from build123d import *

# Parameters (mm, degrees)
BOSS_EXTRUDE1_DEPTH = 19.05
SKETCH2_R           = 3.175
CUT_EXTRUDE1_DEPTH  = 169.2497345
SKETCH4_W           = 25.654
SKETCH4_H           = 25.654
CUT_EXTRUDE2_DEPTH  = 169.2497345


with BuildPart() as part:
    # Sketch1 → Boss-Extrude1 (new body)
    with BuildSketch(Plane(origin=(0, 0, 0), x_dir=(1, 0, 0), z_dir=(0, 1, 0))):
        with BuildLine():
            Line((41.324442937, 92.816218496), (0, 0))
            Line((0, 0), (0, 101.6))
            Line((0, 101.6), (-21.123827787, 99.379796235))
            Line((-21.123827787, 99.379796235), (-26.134113546, 108.80277326))
            ThreePointArc((-26.134113546, 108.80277326), (-30.395027803, 112.639317689), (-36.125160716, 112.83941834))
            Line((-36.125160716, 112.83941834), (-37.099477034, 112.522843778))
            ThreePointArc((-37.099477034, 112.522843778), (-41.617635729, 108.992871331), (-42.809723539, 103.384539126))
            Line((-42.809723539, 103.384539126), (-41.324442937, 92.816218496))
            Line((-41.324442937, 92.816218496), (-59.718981633, 82.196126628))
            Line((-59.718981633, 82.196126628), (-68.128775472, 88.766577677))
            ThreePointArc((-68.128775472, 88.766577677), (-73.58177754, 90.538365452), (-78.897902701, 88.390511467))
            Line((-78.897902701, 88.390511467), (-79.659222473, 87.705016066))
            ThreePointArc((-79.659222473, 87.705016066), (-82.350996682, 82.642525071), (-81.158908872, 77.034192866))
            Line((-81.158908872, 77.034192866), (-75.503514269, 67.983669606))
            Line((-75.503514269, 67.983669606), (-87.988181024, 50.8))
            Line((-87.988181024, 50.8), (-98.343353189, 53.381834395))
            ThreePointArc((-98.343353189, 53.381834395), (-104.04556947, 52.782507313), (-108.028480544, 48.658082159))
            Line((-108.028480544, 48.658082159), (-108.445164665, 47.722194301))
            ThreePointArc((-108.445164665, 47.722194301), (-108.845122174, 42.002535442), (-105.474981556, 37.363934825))
            Line((-105.474981556, 37.363934825), (-96.627342056, 31.396126628))
            Line((-96.627342056, 31.396126628), (-101.043424569, 10.620091868))
            Line((-101.043424569, 10.620091868), (-111.553471718, 8.766886987))
            ThreePointArc((-111.553471718, 8.766886987), (-116.518937215, 5.900074146), (-118.479952693, 0.512228401))
            Line((-118.479952693, 0.512228401), (-118.479952693, -0.512228401))
            ThreePointArc((-118.479952693, -0.512228401), (-116.518937215, -5.900074146), (-111.553471718, -8.766886987))
            Line((-111.553471718, -8.766886987), (-101.043424569, -10.620091868))
            Line((-101.043424569, -10.620091868), (-96.627342056, -31.396126628))
            Line((-96.627342056, -31.396126628), (-105.474981556, -37.363934825))
            ThreePointArc((-105.474981556, -37.363934825), (-108.845122174, -42.002535442), (-108.445164665, -47.722194301))
            Line((-108.445164665, -47.722194301), (-108.028480544, -48.658082159))
            ThreePointArc((-108.028480544, -48.658082159), (-104.04556947, -52.782507313), (-98.343353189, -53.381834395))
            Line((-98.343353189, -53.381834395), (-87.988181024, -50.8))
            Line((-87.988181024, -50.8), (-75.503514269, -67.983669606))
            Line((-75.503514269, -67.983669606), (-81.158908872, -77.034192866))
            ThreePointArc((-81.158908872, -77.034192866), (-82.350996682, -82.642525071), (-79.659222473, -87.705016066))
            Line((-79.659222473, -87.705016066), (-78.897902701, -88.390511467))
            ThreePointArc((-78.897902701, -88.390511467), (-73.58177754, -90.538365452), (-68.128775472, -88.766577677))
            Line((-68.128775472, -88.766577677), (-59.718981633, -82.196126628))
            Line((-59.718981633, -82.196126628), (-41.324442937, -92.816218496))
            Line((-41.324442937, -92.816218496), (-42.809723539, -103.384539126))
            ThreePointArc((-42.809723539, -103.384539126), (-41.617635729, -108.992871331), (-37.099477034, -112.522843778))
            Line((-37.099477034, -112.522843778), (-36.125160716, -112.83941834))
            ThreePointArc((-36.125160716, -112.83941834), (-30.395027803, -112.639317689), (-26.134113546, -108.80277326))
            Line((-26.134113546, -108.80277326), (-21.123827787, -99.379796235))
            Line((-21.123827787, -99.379796235), (0, -101.6))
            Line((0, -101.6), (2.941651908, -111.858759352))
            ThreePointArc((2.941651908, -111.858759352), (6.311792526, -116.497359969), (11.875105022, -117.884449563))
            Line((11.875105022, -117.884449563), (12.893949744, -117.777364667))
            ThreePointArc((12.893949744, -117.777364667), (18.047298371, -115.263908602), (20.379374034, -110.025980903))
            Line((20.379374034, -110.025980903), (21.123827787, -99.379796235))
            Line((21.123827787, -99.379796235), (41.324442937, -92.816218496))
            Line((41.324442937, -92.816218496), (48.184389016, -100.991583882))
            ThreePointArc((48.184389016, -100.991583882), (53.149854513, -103.858396723), (58.796373538, -102.862763072))
            Line((58.796373538, -102.862763072), (59.683579155, -102.35053467))
            ThreePointArc((59.683579155, -102.35053467), (63.369082702, -97.958322577), (63.369082702, -92.224696894))
            Line((63.369082702, -92.224696894), (59.718981633, -82.196126628))
            Line((59.718981633, -82.196126628), (75.503514269, -67.983669606))
            Line((75.503514269, -67.983669606), (85.095607522, -72.662046078))
            ThreePointArc((85.095607522, -72.662046078), (90.797823803, -73.26137316), (95.551214921, -70.055170367))
            Line((95.551214921, -70.055170367), (96.153375521, -69.226367403))
            ThreePointArc((96.153375521, -69.226367403), (97.733776944, -63.714852656), (95.401701281, -58.476924957))
            Line((95.401701281, -58.476924957), (87.988181024, -50.8))
            Line((87.988181024, -50.8), (96.627342056, -31.396126628))
            Line((96.627342056, -31.396126628), (107.293022418, -31.768580394))
            ThreePointArc((107.293022418, -31.768580394), (112.746024485, -29.996792619), (115.784383188, -25.134402274))
            Line((115.784383188, -25.134402274), (115.997379734, -24.13233231))
            ThreePointArc((115.997379734, -24.13233231), (115.199413268, -18.454505879), (110.938499011, -14.617961449))
            Line((110.938499011, -14.617961449), (101.043424569, -10.620091868))
            Line((101.043424569, -10.620091868), (101.043424569, 10.620091868))
            Line((101.043424569, 10.620091868), (110.938499011, 14.617961449))
            ThreePointArc((110.938499011, 14.617961449), (115.199413268, 18.454505879), (115.997379734, 24.13233231))
            Line((115.997379734, 24.13233231), (115.784383188, 25.134402274))
            ThreePointArc((115.784383188, 25.134402274), (112.746024485, 29.996792619), (107.293022418, 31.768580394))
            Line((107.293022418, 31.768580394), (96.627342056, 31.396126628))
            Line((96.627342056, 31.396126628), (87.988181024, 50.8))
            Line((87.988181024, 50.8), (95.401701281, 58.476924957))
            ThreePointArc((95.401701281, 58.476924957), (97.733776944, 63.714852656), (96.153375521, 69.226367403))
            Line((96.153375521, 69.226367403), (95.551214921, 70.055170367))
            ThreePointArc((95.551214921, 70.055170367), (90.797823803, 73.26137316), (85.095607522, 72.662046078))
            Line((85.095607522, 72.662046078), (75.503514269, 67.983669606))
            Line((75.503514269, 67.983669606), (59.718981633, 82.196126628))
            Line((59.718981633, 82.196126628), (63.369082702, 92.224696894))
            ThreePointArc((63.369082702, 92.224696894), (63.369082702, 97.958322577), (59.683579155, 102.35053467))
            Line((59.683579155, 102.35053467), (58.796373538, 102.862763072))
            ThreePointArc((58.796373538, 102.862763072), (53.149854513, 103.858396723), (48.184389016, 100.991583882))
            Line((48.184389016, 100.991583882), (41.324442937, 92.816218496))
        make_face()
        with BuildLine():
            Line((0, 101.6), (0, 0))
            Line((0, 0), (21.123827787, 99.379796235))
            Line((21.123827787, 99.379796235), (20.379374034, 110.025980903))
            ThreePointArc((20.379374034, 110.025980903), (18.047298371, 115.263908602), (12.893949744, 117.777364667))
            Line((12.893949744, 117.777364667), (11.875105022, 117.884449563))
            ThreePointArc((11.875105022, 117.884449563), (6.311792526, 116.497359969), (2.941651908, 111.858759352))
            Line((2.941651908, 111.858759352), (0, 101.6))
        make_face()
        Polygon((21.123827787, 99.379796235), (0, 0), (41.324442937, 92.816218496), align=None)
    extrude(amount=BOSS_EXTRUDE1_DEPTH)

    # Sketch2 → Cut-Extrude1 (cut, through all)
    with BuildSketch(Plane(origin=(0, 19.05, 0), x_dir=(1, 0, 0), z_dir=(0, 1, 0))):
        with Locations(Location((0, 0, 0), (0, 0, 270))):
            Circle(SKETCH2_R)
    extrude(amount=-CUT_EXTRUDE1_DEPTH, mode=Mode.SUBTRACT)

    # Sketch4 → Cut-Extrude2 (cut, through all)
    with BuildSketch(Plane(origin=(0, 19.05, 0), x_dir=(1, 0, 0), z_dir=(0, 1, 0))):
        Rectangle(SKETCH4_W, SKETCH4_H)
    extrude(amount=-CUT_EXTRUDE2_DEPTH, mode=Mode.SUBTRACT)


solid = part.part
Geometry: final body of the model. Coordinates: model frame, mm. A direction names the side the tool comes from. Coordinates: 2 decimals unless noted, no trailing zeros. Loops run counter-clockwise (first coordinate to the right, second up) from the corner with the lowest first, then second, coordinate; pieces in that order, holes last. Notation, with made-up numbers: (38, -18.5) - (63, -18.5) arc R29 cw to (63, 5.5) - close; hole circle Ø6 at (62.5, 74). An arc over 180 degrees is marked (long way). One line per question, with ' | ' between items. Start each with the question number.
(1) Draft query along X for faces 1 (the flat face through (80.367, 9.392, -70.356)), 2 (the cylindrical face through (53.069, 9.392, 103.844)), 3 (the cylindrical face through (-41.574, 9.392, -109.062)), 4 (the cylindrical face through (115.24, 9.39, 18.53)). Return one class per face: +X half, -X half, draft (parallel to the pull), parting line (faces both ways), or undercut.
(2) First-contact query: pin 1 (1.5 mm diameter, centred on x = -71, y = 5, fed in from -Z); pin 2 (5.5 mm diameter, centred on x = 0.5, y = 13.5, fed in from +Z); pin 3 (8 mm diameter, centred on y = 11.5, z = 64, fed in from +X). Flat tips, straight axial feed; report the tip coordinate or a pass-through.
(3) Cut plane A-A on x = -52. Output: boundary loops of the cut face in (y, z), and give its area (3 significant figures).
(4) Ray query, L1, parallel to X at y = 6.75, z = -1; L2, parallel to Z at x = -6, y = 14; L3, parallel to Z at x = 92, y = 9. Return the intervals inside material, ascending. Write a range as from..to.
(5) Reachability of faces 5 (the flat face through (80.23, 9.39, 70.29)), 6 (the flat face through (-106.225, 9.392, -9.706)), 7 (the flat face through (31.37, 9.39, -96.05)) from +Z, -Z, +X, -X, +Y, -Y: full face, straight path, thin tool, end or side. Return the list, or none.
(6) Cut plane B-B on z = -65. Output: boundary loops of the cut face in (x, y), and give its area (3 significant figures).
Here are the results:
1) face 1: undercut | face 2: undercut | face 3: -X half | face 4: +X half
2) pin 1: z = -90.4 | pin 2: z = 112.74 | pin 3: x = 97.75
3) outline: (0, -86.65) - (19.05, -86.65) - (19.05, 86.65) - (0, 86.65) - close | area: 3,300 mm²
4) L1: -118.47..-12.83, 12.83..101.04 | L2: -100.97..-12.83, 12.83..100.97 | L3: -72.86..-54.95, -41.79..41.79, 54.95..72.86
5) face 5: +Z, +Y, -Y | face 6: -X, +Y, -Y | face 7: -Z, +Y, -Y
6) outline: (-77.67, 0) - (97.72, 0) - (97.72, 19.05) - (-77.67, 19.05) - close | area: 3,340 mm²
